```python
from build123d import *

# Parameters (mm, degrees)
SKETCH1_W           = 30
SKETCH1_H           = 14
BOSS_EXTRUDE1_DEPTH = 7.2
SKETCH2_R           = 0.225
BOSS_EXTRUDE2_DEPTH = 8


with BuildPart() as part:
    # Sketch1 → Boss-Extrude1 (new body)
    with BuildSketch(Plane(origin=(0, 0, 0), x_dir=(1, 0, 0), z_dir=(0, 1, 0))):
        Rectangle(SKETCH1_W, SKETCH1_H)
    extrude(amount=BOSS_EXTRUDE1_DEPTH)

    # Sketch2 → Boss-Extrude2 (add)
    with BuildSketch(Plane.XZ):
        with Locations(Location((-6.35, -5.08, 0), (0, 0, 270))):
            Circle(SKETCH2_R)
        with Locations(Location((-3.81, -5.08, 0), (0, 0, 270))):
            Circle(SKETCH2_R)
        with Locations(Location((-1.27, -5.08, 0), (0, 0, 270))):
            Circle(SKETCH2_R)
        with Locations(Location((1.27, -5.08, 0), (0, 0, 270))):
            Circle(SKETCH2_R)
        with Locations(Location((3.81, -5.08, 0), (0, 0, 270))):
            Circle(SKETCH2_R)
        with Locations(Location((6.35, -5.08, 0), (0, 0, 270))):
            Circle(SKETCH2_R)
        with Locations(Location((-3.81, 5.08, 0), (0, 0, 270))):
            Circle(SKETCH2_R)
        with Locations(Location((-1.27, 5.08, 0), (0, 0, 270))):
            Circle(SKETCH2_R)
        with Locations(Location((1.27, 5.08, 0), (0, 0, 270))):
            Circle(SKETCH2_R)
        with Locations(Location((3.81, 5.08, 0), (0, 0, 270))):
            Circle(SKETCH2_R)
        with Locations(Location((6.35, 5.08, 0), (0, 0, 270))):
            Circle(SKETCH2_R)
        with Locations(Location((-6.35, 5.08, 0), (0, 0, 270))):
            Circle(SKETCH2_R)
    extrude(amount=BOSS_EXTRUDE2_DEPTH)


solid = part.part
```
For this review, take the finished solid that the model builds, in its own axes (mm). Coordinates: 2 decimals unless noted, no trailing zeros. Write each loop counter-clockwise with the first axis right and the second up, starting at its lowest first coordinate (ties: lowest second). Pieces come first, ordered by that corner, then holes. Notation, with made-up numbers: (22.5, 30) - (69.5, 30) arc R27 cw to (69.5, 66) - close; hole circle Ø2 at (-18.5, -24.5). An arc over 180 degrees is marked (long way). Put each result on its own line as item: value.
1. For pin 1 (4 mm diameter, centred on x = -3, y = -6, fed in from +Z) (3 decimals); pin 2 (6 mm diameter, centred on x = 9, z = -1.5, fed in from -Y), all flat-tipped, find the tip position at first contact; note any pin that passes through.
Values found:
pin 1: z = 5.305
pin 2: y = 0
2. Wall thickness on probe 1 along Y at (x, z) = (9, -5.25); probe 2 along Z at (x, y) = (1.25, -6.75): over which ranges is each line inside the solid? List them lowest first.
Values found:
probe 1: 0 to 7.2
probe 2: -5.3 to -4.86, 4.86 to 5.3
3. Add section C-C, the plane x = 11.5. Give the boundary of the cut face in (y, z).
Values found:
outline: (0, -7) - (7.2, -7) - (7.2, 7) - (0, 7) - close
4. Add section B-B, the plane z = 4. Give the boundary of the cut face in (x, y).
Values found:
outline: (-15, 0) - (15, 0) - (15, 7.2) - (-15, 7.2) - close
5. Add section A-A, the plane y = -4.5. Count the separate pieces of the cut face and the enclosed holes in it, then the cut area to 3 significant figures.
Values found:
separate pieces: 12
enclosed holes: 0
area: 1.91 mm²
